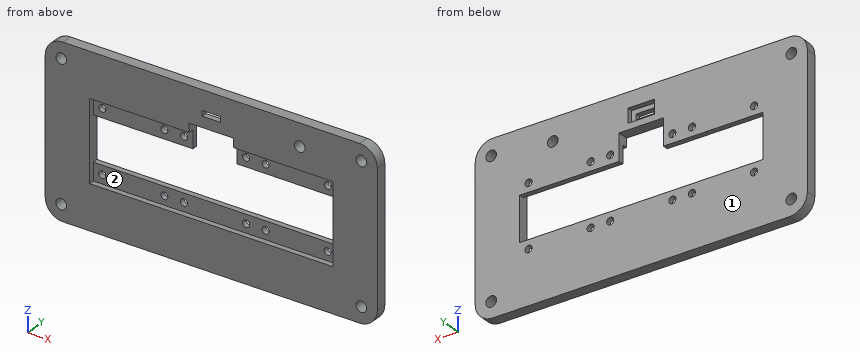
from build123d import *

# Parameters (mm, degrees)
F0_W     = 187
F0_H     = 95
F0_R     = 3
F0_W_2   = 10.25
F0_H_2   = 3
F1_DEPTH = 6
F2_R     = 10
F3_W     = 15
F3_H     = 8
F4_DEPTH = 3
F5_R     = 2
F6_DEPTH = 3


with BuildPart() as f1:
    # F0 (on Front) → F1 (new body)
    with BuildSketch(Plane.XZ):
        Rectangle(F0_W, F0_H)
        with Locations((-84.5, -38.5)):
            Circle(F0_R, mode=Mode.SUBTRACT)
        with Locations((84.5, -38.5)):
            Circle(F0_R, mode=Mode.SUBTRACT)
        Polygon((12.5, 22.5), (68.5, 22.5), (68.5, -22.5), (-68.5, -22.5), (-68.5, 22.5), (-12.5, 22.5), (-12.5, 27.5), (12.5, 27.5), align=None, mode=Mode.SUBTRACT)
        with Locations((-84.5, 38.5)):
            Circle(F0_R, mode=Mode.SUBTRACT)
        with Locations((0, 35)):
            Rectangle(F0_W_2, F0_H_2, mode=Mode.SUBTRACT)
        with Locations((49.831439, 35)):
            Circle(F0_R, mode=Mode.SUBTRACT)
        with Locations((84.5, 38.5)):
            Circle(F0_R, mode=Mode.SUBTRACT)
    extrude(amount=F1_DEPTH)

    # F2
    f2_edges = [f1.edges().sort_by_distance(p)[0] for p in [
        (93.5, -3, -47.5),
        (-93.5, -3, -47.5),
        (-93.5, -3, 47.5),
        (93.5, -3, 47.5),
    ]]
    fillet(f2_edges, radius=F2_R)

    # F3 (on face) → F4 (cut)
    with BuildSketch(Plane(origin=(0, 0, 0), x_dir=(-1, 0, 0), z_dir=(0, 1, 0))):
        with Locations((0, 35)):
            Rectangle(F3_W, F3_H)
    extrude(amount=-F4_DEPTH, mode=Mode.SUBTRACT)

    # F5 (on face) → F6 (join)
    with BuildSketch(Plane(origin=(0, 0, 0), x_dir=(-1, 0, 0), z_dir=(0, 1, 0))):
        Polygon((-12.5, 12.5), (-12.5, 22.5), (-12.5, 27.5), (-75.93517, 27.851377), (-75.93517, 12.5), (-68.5, 12.5), align=None)
        with Locations((-63.5, 17.5)):
            Circle(F5_R, mode=Mode.SUBTRACT)
        with Locations((-28.5, 17.5)):
            Circle(F5_R, mode=Mode.SUBTRACT)
        with Locations((-17.5, 17.5)):
            Circle(F5_R, mode=Mode.SUBTRACT)
        Polygon((71.986005, 27.851377), (12.5, 22.5), (12.5, 12.5), (71.986005, 12.5), align=None)
        with Locations((17.5, 17.5)):
            Circle(F5_R, mode=Mode.SUBTRACT)
        with Locations((28.5, 17.5)):
            Circle(F5_R, mode=Mode.SUBTRACT)
        with Locations((63.5, 17.5)):
            Circle(F5_R, mode=Mode.SUBTRACT)
        Polygon((72.550595, -12.5), (-68.5, -12.5), (-73.253393, -11.935415), (-76.499753, -24.073985), (72.550595, -24.073985), align=None)
        with Locations((-63.5, -17.5)):
            Circle(F5_R, mode=Mode.SUBTRACT)
        with Locations((-28.5, -17.5)):
            Circle(F5_R, mode=Mode.SUBTRACT)
        with Locations((-17.5, -17.5)):
            Circle(F5_R, mode=Mode.SUBTRACT)
        with Locations((17.5, -17.5)):
            Circle(F5_R, mode=Mode.SUBTRACT)
        with Locations((28.5, -17.5)):
            Circle(F5_R, mode=Mode.SUBTRACT)
        with Locations((63.5, -17.5)):
            Circle(F5_R, mode=Mode.SUBTRACT)
    extrude(amount=-F6_DEPTH)


solid = f1.part
Build history of the part. All positions in model axes, mm. Face numbers are marked on the shaded views. Coordinates: 2 decimals unless noted, no trailing zeros. Order: outer loops, then holes, each group sorted by start corner. A loop starts at its lowest first (then second) coordinate and runs counter-clockwise, first axis right, second up. Notation, with made-up numbers: M -22.5,-27 L -8.5,-27 A18 ccw -8.5,-6 Z; hole C -20,70 d9. An arc over 180 degrees is marked long. One line per question, with ' | ' between items. Start each with the question number.
Q1. Flat gauge pins, fed straight in: pin 1 Ø3 at (x, z) = (28.5, 17.5) entering from +Y; pin 2 Ø5 at (x, z) = (-17.5, 17.5) entering from -Y; pin 3 Ø4 at (x, z) = (2, 35.5) entering from +Y; pin 4 Ø7 at (x, z) = (-84.5, -38.5) entering from -Y. Where does each tip first touch, or does it go through?
Q2. Probe L1, parallel to Z at x = -28.5, y = -1.8; L2, parallel to X at y = -0.3, z = -5.5; L3, parallel to Z at x = 43, y = -5. List the from-to ranges inside material, lowest first. Write a range as from..to.
Q3. Saw through at B-B (z = -17.5). Count the separate pieces of the cut face and the enclosed holes in it, then the cut area to 3 significant figures.
Q4. Saw through at C-C (y = -3.9). List the corners of the cut face in (x, z) (3 decimals).
Q5. Saw through at A-A (x = -55.5). List the corners of the cut face in (y, z).
Q6. Two-plate mould, pull along Z, no slides. Class the marked faces 1 and 2: +Z half, -Z half, draft (parallel to the pull), parting line (faces both ways), or undercut.
Check values:
1) pin 1: passes through | pin 2: stops at y = -3 | pin 3: stops at y = -3 | pin 4: stops at y = -6
2) L1: z = -47.5..-19.5, -15.5..-12.5, 12.5..15.5, 19.5..47.5 | L2: x = -93.5..-68.5, 68.5..93.5 | L3: z = -47.5..-22.5, 22.5..47.5
3) separate pieces: 7 | enclosed holes: 0 | area: 639 mm2
4) outline: M -93.5,-37.5 A10 ccw -83.5,-47.5 L 83.5,-47.5 A10 ccw 93.5,-37.5 L 93.5,37.5 A10 ccw 83.5,47.5 L -83.5,47.5 A10 ccw -93.5,37.5 Z; hole C -84.5,-38.5 d6; hole C -84.5,38.5 d6; hole M -68.5,-22.5 L 68.5,-22.5 L 68.5,22.5 L 12.5,22.5 L 12.5,27.5 L -12.5,27.5 L -12.5,22.5 L -68.5,22.5 Z; hole M -5.125,33.5 L 5.125,33.5 L 5.125,36.5 L -5.125,36.5 Z; hole C 49.831,35 d6; hole C 84.5,-38.5 d6; hole C 84.5,38.5 d6
5) outline: M -6,-47.5 L 0,-47.5 L 0,-12.5 L -3,-12.5 L -3,-22.5 L -6,-22.5 Z; M -6,22.5 L -3,22.5 L -3,12.5 L 0,12.5 L 0,47.5 L -6,47.5 Z
6) face 1: draft | face 2: undercut
